For this review, take the finished solid that the model builds, in its own axes (mm). Round coordinates to 2 decimals unless told otherwise and drop trailing zeros. Loops run counter-clockwise (first coordinate to the right, second up) from the corner with the lowest first, then second, coordinate; pieces in that order, holes last. Notation, with made-up numbers: (78, 15) -> (86, 15) arc R22 ccw to (86, 38) -> close; hole circle Ø9 at (-30, 21.5). An arc over 180 degrees is marked (long way). One line per question, with ' | ' between items. Start each with the question number.
1. For pin 1 Ø3 at (x, z) = (130.71, -54.95) entering from -Y, flat-tipped, find the tip position at first contact; note if it passes through.
2. Draft analysis for pull direction X (two halves, no side actions). For faces 1 (the face through (156.38, 1.77, -55.48)), 2 (the face through (94, 0, -86)), 3 (the face through (30.088, 1.825, -33.007)), state which applies: pulls with the +X half, pulls with the -X half, needs draft (parallel to the pull), parting line crosses it, or undercut.
3. Consider section A-A (z = -54.95). Write out the cut boundary in (x, y).
4. Wall thickness on line 1 along X through (y, z) = (0.9, -54.95); line 2 along Z through (x, y) = (76, 0.65); line 3 along Z through (x, y) = (34, 2.65): over which ranges is each line inside the solid? List them lowest first.
5. Consider section C-C (z = -132). Write out the cut boundary in (x, y).
6. Consider section B-B (x = 76.2). Write out the cut boundary in (y, z), and give its area (3 significant figures).
```python
from build123d import *

# Parameters (mm, degrees)
SKETCH_6_W      = 135.527465206
SKETCH_6_H      = 109.875291841
SKETCH_6_R      = 1.75
SKETCH_6_R_2    = 1.5
EXTRUDE_2_DEPTH = 3.6
FILLET_1_R      = 10
FILLET_2_R      = 10
FILLET_3_R      = 10
FILLET_4_R      = 10


with BuildPart() as part:
    # 草图6 → 凸台-拉伸2 (new body)
    with BuildSketch(Plane(origin=(0, 0, 0), x_dir=(1, 0, 0), z_dir=(0, 1, 0))):
        with Locations((95, 84.937645921)):
            Rectangle(SKETCH_6_W, SKETCH_6_H)
        with Locations((35.286267397, 54.95)):
            Circle(SKETCH_6_R, mode=Mode.SUBTRACT)
        with Locations((59.286267397, 54.95)):
            Circle(SKETCH_6_R, mode=Mode.SUBTRACT)
        with Locations((35.286267397, 85.05)):
            Circle(SKETCH_6_R, mode=Mode.SUBTRACT)
        with Locations((59.286267397, 85.05)):
            Circle(SKETCH_6_R, mode=Mode.SUBTRACT)
        with Locations((76.2, 132)):
            Circle(SKETCH_6_R_2, mode=Mode.SUBTRACT)
        with Locations((113.8, 132)):
            Circle(SKETCH_6_R_2, mode=Mode.SUBTRACT)
        with Locations((130.713732603, 85.05)):
            Circle(SKETCH_6_R, mode=Mode.SUBTRACT)
        with Locations((154.713732603, 54.95)):
            Circle(SKETCH_6_R, mode=Mode.SUBTRACT)
        with Locations((154.713732603, 85.05)):
            Circle(SKETCH_6_R, mode=Mode.SUBTRACT)
        with Locations((130.713732603, 54.95)):
            Circle(SKETCH_6_R, mode=Mode.SUBTRACT)
    extrude(amount=EXTRUDE_2_DEPTH)

    # 圆角1
    fillet_1_edges = [part.edges().sort_by_distance(p)[0] for p in [
        (27.236267397, 1.8, -30),
    ]]
    fillet(fillet_1_edges, radius=FILLET_1_R)

    # 圆角2
    fillet_2_edges = [part.edges().sort_by_distance(p)[0] for p in [
        (27.236267397, 1.8, -139.875291841),
    ]]
    fillet(fillet_2_edges, radius=FILLET_2_R)

    # 圆角3
    fillet_3_edges = [part.edges().sort_by_distance(p)[0] for p in [
        (162.763732603, 1.8, -139.875291841),
    ]]
    fillet(fillet_3_edges, radius=FILLET_3_R)

    # 圆角4
    fillet_4_edges = [part.edges().sort_by_distance(p)[0] for p in [
        (162.763732603, 1.8, -30),
    ]]
    fillet(fillet_4_edges, radius=FILLET_4_R)


solid = part.part
```
Answer block:
1) pin 1: passes through
2) face 1: undercut | face 2: needs draft | face 3: pulls with the -X half
3) outline: (27.24, 0) -> (33.54, 0) -> (33.54, 3.6) -> (27.24, 3.6) -> close; (37.04, 0) -> (57.54, 0) -> (57.54, 3.6) -> (37.04, 3.6) -> close; (61.04, 0) -> (128.96, 0) -> (128.96, 3.6) -> (61.04, 3.6) -> close; (132.46, 0) -> (152.96, 0) -> (152.96, 3.6) -> (132.46, 3.6) -> close; (156.46, 0) -> (162.76, 0) -> (162.76, 3.6) -> (156.46, 3.6) -> close
4) line 1: x = 27.24 to 33.54, 37.04 to 57.54, 61.04 to 128.96, 132.46 to 152.96, 156.46 to 162.76 | line 2: z = -139.88 to -133.49, -130.51 to -30 | line 3: z = -139.34 to -86.24, -83.86 to -56.14, -53.76 to -30.54
5) outline: (27.46, 0) -> (74.7, 0) -> (74.7, 3.6) -> (27.46, 3.6) -> close; (77.7, 0) -> (112.3, 0) -> (112.3, 3.6) -> (77.7, 3.6) -> close; (115.3, 0) -> (162.54, 0) -> (162.54, 3.6) -> (115.3, 3.6) -> close
6) outline: (0, -139.88) -> (3.6, -139.88) -> (3.6, -133.5) -> (0, -133.5) -> close; (0, -130.5) -> (3.6, -130.5) -> (3.6, -30) -> (0, -30) -> close | area: 385 mm2
